Model file for the job. Use its own axes, mm. Round coordinates to 2 decimals unless told otherwise and drop trailing zeros. Loops run counter-clockwise (first coordinate to the right, second up) from the corner with the lowest first, then second, coordinate; pieces in that order, holes last. Notation, with made-up numbers: (62, 57.5) - (79, 57.5) arc R36 ccw to (79, 96.5) - close; hole circle Ø3 at (-8.5, -35). An arc over 180 degrees is marked (long way). Answer as a JSON object with one key per item and string values.
Autodesk Inventor part; units mm, degrees
ref_plane "YZ Plane" through (0, 0, 0) normal (1, 0, 0) x (0, 1, 0)
ref_plane "XZ Plane" through (0, 0, 0) normal (0, 1, 0) x (-1, 0, 0)
ref_plane "XY Plane" through (0, 0, 0) normal (0, 0, 1) x (1, 0, 0)
sketch "スケッチ1" plane through (0, 0, 0) normal (0, 0, 1) x (1, 0, 0)
  line L0 (0, 0) -> (15, 0)
  line L1 (15, 0) -> (15, 15)
  line L2 (15, 15) -> (0, 15)
  line L3 (0, 15) -> (0, 0)
  circle A0 centre (7.5, 7.5) radius 4
  line L4 (15, 15) -> (25, 15)
  line L5 (25, 15) -> (25, 0)
  line L6 (25, 0) -> (15, 0)
  line L7 (15, 0) -> (15, 15)
  circle A1 centre (20, 12.5) radius 1.5
  circle A2 centre (20, 2.5) radius 1.5
  dimension "d0" = 15
  dimension "d1" = 15
  dimension "d2" = 8
  dimension "d3" = 7.5
  dimension "d4" = 7.5
  dimension "d5" = 10
  dimension "d6" = 10
  dimension "d7" = 2.5
  dimension "d8" = 2.5
  dimension "d9" = 3
  dimension "d10" = 3
extrude "押し出し1" add sketch "スケッチ1" along normal blind 2
fillet "フィレット1" radius 2 4 edges at (0, 15, 1) (0, 0, 1) (25, 0, 1) (25, 15, 1)
equation "\"d1\" = d0"
equation "\"d4\" = 0.5 * d1"
properties part number "finger_al_mk_1" material "アルミニウム 6061-AHC"
1) Slice it at D-D on x = 9. List the corners of the cut face in (y, z), then the cut area to 3 significant figures.
Values follow:
{"outline": "(0, 0) - (3.79, 0) - (3.79, 2) - (0, 2) - close; (11.21, 0) - (15, 0) - (15, 2) - (11.21, 2) - close", "area": "15.2 mm²"}
2) Drop a flat-ended pin along its axis: P1, Ø5, axis at x = 7.5, y = 7.5, coming from the +Z side. Give the stop position or say it passes through.
Values follow:
{"P1": "through"}
3) Two-plate mould, pull along X, no slides. Class faces 1 (the cylindrical face through (3.504, 7.324, 0.986)), 2 (the cylindrical face through (18.5, 2.43, 0.99)), 3 (the flat face through (0, 8, 1)), 4 (the flat face through (12, 8, 2)): pulls with the +X half, pulls with the -X half, needs draft (parallel to the pull), parting line crosses it, or undercut.
Values follow:
{"face 1": "undercut", "face 2": "undercut", "face 3": "pulls with the -X half", "face 4": "needs draft"}
4) Slice it at A-A on y = 7.5. List the corners of the cut face in (x, z), then the cut area to 3 significant figures.
Values follow:
{"outline": "(0, 0) - (3.5, 0) - (3.5, 2) - (0, 2) - close; (11.5, 0) - (25, 0) - (25, 2) - (11.5, 2) - close", "area": "34.0 mm²"}
5) Probe probe 1 along Y at (x, z) = (20, 0.5); probe 2 along Y at (x, z) = (21, 1.7); probe 3 along X at (y, z) = (12.75, 1.4). List the from-to ranges inside material, lowest first.
Values follow:
{"probe 1": "0 to 1, 4 to 11, 14 to 15", "probe 2": "0 to 1.38, 3.62 to 11.38, 13.62 to 15", "probe 3": "0 to 18.52, 21.48 to 25"}
6) Slice it at C-C on z = 1.25. List the corners of the cut face in (x, y), then the cut area to 3 significant figures.
Values follow:
{"outline": "(0, 2) arc R2 ccw to (2, 0) - (23, 0) arc R2 ccw to (25, 2) - (25, 13) arc R2 ccw to (23, 15) - (2, 15) arc R2 ccw to (0, 13) - close; hole circle Ø8 at (7.5, 7.5); hole circle Ø3 at (20, 2.5); hole circle Ø3 at (20, 12.5)", "area": "307 mm²"}
7) Slice it at B-B on x = 20. List the corners of the cut face in (y, z).
Values follow:
{"outline": "(0, 0) - (1, 0) - (1, 2) - (0, 2) - close; (4, 0) - (11, 0) - (11, 2) - (4, 2) - close; (14, 0) - (15, 0) - (15, 2) - (14, 2) - close"}
